Source: CAD feature listing. Evaluate the final solid. Frame: model axes, mm. A direction names the side the tool comes from. Give positions to 0.01 mm unless a question says otherwise; leave off trailing zeros. Write each loop counter-clockwise with the first axis right and the second up, starting at its lowest first coordinate (ties: lowest second). Pieces come first, ordered by that corner, then holes. Notation, with made-up numbers: M 80,4 L 114,4 A26 ccw 114,20 Z; hole C -18.5,15.5 d10. An arc over 180 degrees is marked long. Return JSON: item names as keys, results as strings.
```python
from build123d import *

# Parameters (mm, degrees)
SKETCH_1_W          = 25
SKETCH_1_H          = 70
SKETCH_1_R          = 1.3
SKETCH_1_R_2        = 1.65
EXTRUDE_1_DEPTH     = 5
SKETCH_2_R          = 2.9
CUT_EXTRUDE_1_DEPTH = 3.2
CUT_EXTRUDE_2_DEPTH = 3.2
FILLET_1_R          = 1.5
EXTRUDE_2_DEPTH     = 3


with BuildPart() as part:
    # 草图1 → 凸台-拉伸1 (new body)
    with BuildSketch(Plane(origin=(0, 0, 0), x_dir=(1, 0, 0), z_dir=(0, 1, 0))):
        Rectangle(SKETCH_1_W, SKETCH_1_H)
        with Locations((10, 25)):
            Circle(SKETCH_1_R, mode=Mode.SUBTRACT)
        with Locations((10, 0)):
            Circle(SKETCH_1_R, mode=Mode.SUBTRACT)
        with Locations((10, -25)):
            Circle(SKETCH_1_R, mode=Mode.SUBTRACT)
        with Locations((0, 23)):
            Circle(SKETCH_1_R_2, mode=Mode.SUBTRACT)
        with Locations((0, -23)):
            Circle(SKETCH_1_R_2, mode=Mode.SUBTRACT)
        with Locations((-10, 25)):
            Circle(SKETCH_1_R, mode=Mode.SUBTRACT)
        with Locations((-10, 0)):
            Circle(SKETCH_1_R, mode=Mode.SUBTRACT)
        with Locations((-10, -25)):
            Circle(SKETCH_1_R, mode=Mode.SUBTRACT)
    extrude(amount=EXTRUDE_1_DEPTH)

    # 草图2 → 切除-拉伸1 (cut)
    with BuildSketch(Plane(origin=(0, 5, 0), x_dir=(1, 0, 0), z_dir=(0, 1, 0))):
        with Locations((0, 23)):
            Circle(SKETCH_2_R)
        with Locations((0, -23)):
            Circle(SKETCH_2_R)
    extrude(amount=-CUT_EXTRUDE_1_DEPTH, mode=Mode.SUBTRACT)

    # 草图3 → 切除-拉伸2 (cut)
    with BuildSketch(Plane.XZ):
        Polygon((-7.375, 23.484455543), (-7.375, 26.515544457), (-10, 28.031088913), (-12.625, 26.515544457), (-12.625, 23.484455543), (-10, 21.968911087), align=None)
        Polygon((10, 28.031088913), (7.375, 26.515544457), (7.375, 23.484455543), (10, 21.968911087), (12.625, 23.484455543), (12.625, 26.515544457), align=None)
        Polygon((10, 3.031088913), (7.375, 1.515544457), (7.375, -1.515544457), (10, -3.031088913), (12.625, -1.515544457), (12.625, 1.515544457), align=None)
        Polygon((-10, 3.031088913), (-12.625, 1.515544457), (-12.625, -1.515544457), (-10, -3.031088913), (-7.375, -1.515544457), (-7.375, 1.515544457), align=None)
        Polygon((-7.375, -26.515544457), (-7.375, -23.484455543), (-10, -21.968911087), (-12.625, -23.484455543), (-12.625, -26.515544457), (-10, -28.031088913), align=None)
        Polygon((10, -21.968911087), (7.375, -23.484455543), (7.375, -26.515544457), (10, -28.031088913), (12.625, -26.515544457), (12.625, -23.484455543), align=None)
    extrude(amount=-CUT_EXTRUDE_2_DEPTH, mode=Mode.SUBTRACT)

    # 圆角1
    fillet_1_edges = [part.edges().sort_by_distance(p)[0] for p in [
        (12.5, 2.5, 35),
        (-12.5, 2.5, 35),
        (-12.5, 2.5, -35),
        (12.5, 2.5, -35),
    ]]
    fillet(fillet_1_edges, radius=FILLET_1_R)

    # 草图4 → 凸台-拉伸2 (add, symmetric)
    with BuildSketch(Plane(origin=(0, 0, 0), x_dir=(0, 0, -1), z_dir=(1, 0, 0))):
        Polygon((-34, 0), (-27, 0), (-29, -2), (-32, -2), align=None)
        Polygon((29, -2), (32, -2), (34, 0), (27, 0), align=None)
    extrude(amount=EXTRUDE_2_DEPTH, both=True)


solid = part.part
```
1) Cut plane B-B, the plane z = 0. Return the cut outline in (x, y) (3 decimals).
Numbers:
{"outline": "M -12.5,3.2 L -11.3,3.2 L -11.3,5 L -12.5,5 Z; M -8.7,3.2 L -7.375,3.2 L -7.375,0 L 7.375,0 L 7.375,3.2 L 8.7,3.2 L 8.7,5 L -8.7,5 Z; M 11.3,3.2 L 12.5,3.2 L 12.5,5 L 11.3,5 Z"}
2) Cut plane A-A, the plane x = 0. Return the cut outline in (y, z).
Numbers:
{"outline": "M -2,-32 L 0,-34 L 0,-35 L 5,-35 L 5,-25.9 L 1.8,-25.9 L 1.8,-24.65 L 0,-24.65 L 0,-27 L -2,-29 Z; M -2,29 L 0,27 L 0,24.65 L 1.8,24.65 L 1.8,25.9 L 5,25.9 L 5,35 L 0,35 L 0,34 L -2,32 Z; M 0,-21.35 L 1.8,-21.35 L 1.8,-20.1 L 5,-20.1 L 5,20.1 L 1.8,20.1 L 1.8,21.35 L 0,21.35 Z"}
3) Line query: line 1 (Z direction, x = 7.5, y = 1); line 2 (Z direction, x = -10, y = 4); line 3 (X direction, y = 4.5, z = -25). Output: solid intervals per line, ascending. Write a range as [from, to].
Numbers:
{"line 1": "z = [-35, -26.59], [-23.41, -1.59], [1.59, 23.41], [26.59, 35]", "line 2": "z = [-35, -26.3], [-23.7, -1.3], [1.3, 23.7], [26.3, 35]", "line 3": "x = [-12.5, -11.3], [-8.7, -2.1], [2.1, 8.7], [11.3, 12.5]"}
4) Cut plane D-D, the plane z = -31. Return the cut outline in (x, y), then the cut area to 3 significant figures.
Numbers:
{"outline": "M -12.5,0 L -3,0 L -3,-2 L 3,-2 L 3,0 L 12.5,0 L 12.5,5 L -12.5,5 Z", "area": "137 mm²"}
5) Contact query for flat-ended pins moving along their axis: pin 1 Ø3.5 at (y, z) = (1.5, 24.5) entering from +X; pin 2 Ø5.5 at (x, z) = (9.5, -24.5) entering from -Y; pin 3 Ø2.5 at (y, z) = (1.5, -25) entering from +X (3 decimals); pin 4 Ø3.5 at (x, z) = (10, 0) entering from -Y. Output: stop coordinate, or through.
Numbers:
{"pin 1": "stops at x = 12.5", "pin 2": "stops at y = 0", "pin 3": "stops at x = 7.375", "pin 4": "stops at y = 3.2"}
6) Cut plane C-C, the plane y = 4.25. Give the number of separate pieces and of enclosed holes in the cut face, then the cut area to 3 significant figures.
Numbers:
{"separate pieces": "1", "enclosed holes": "8", "area": "1,660 mm²"}
7) Draft query along X for faces 4 (the face through (-7.375, 2, 0)), 5 (the face through (12.05, 2.54, 34.57)), 6 (the face through (-8.669, 1.578, -22.737)). Return one class per face: released by +X, released by -X, zero draft, split by the parting line, or undercut.
Numbers:
{"face 4": "released by -X", "face 5": "released by +X", "face 6": "undercut"}
8) Set-up query: faces 1 (the face through (7.375, 2, -25)), 2 (the face through (-3, -1, 30)), 3 (the face through (9.3, 3.2, 23.7)). Return all of +Z, -Z, +X, -X, +Y, -Y with unobstructed straight access to the full face (end or side cutting, diameter ignored); none if empty.
Numbers:
{"face 1": "+X, -Y", "face 2": "+Z, -Z, -X, -Y", "face 3": "-Y"}
